```python
from build123d import *

# Parameters (mm, degrees)
SKETCH_R          = 29
PAD_DEPTH         = 35
SKETCH001_W       = 5
SKETCH001_H       = 16
PAD001_DEPTH      = 20
SKETCH002_R       = 4
PAD002_DEPTH      = 66
PAD002_DEPTH_BACK = 48
SKETCH003_R       = 4
SKETCH003_R_2     = 2.4
POCKET_DEPTH      = 20
SKETCH004_R       = 3.25
POCKET001_DEPTH   = 5
FILLET_R          = 2
FILLET001_R       = 7.5


with BuildPart() as part:
    # Sketch → Pad (new body)
    with BuildSketch(Plane.XY):
        Circle(SKETCH_R)
    extrude(amount=PAD_DEPTH)

    # Sketch001 (on Face2 of Pad) → Pad001 (join)
    with BuildSketch(Plane(origin=(0, 0, 0), x_dir=(1, 0, 0), z_dir=(0, 0, -1))):
        Rectangle(SKETCH001_W, SKETCH001_H)
    extrude(amount=PAD001_DEPTH)

    # Sketch002 → Pad002 (join, two sides)
    with BuildSketch(Plane.XZ) as pad002_sk:
        with Locations((0, 8.5)):
            Circle(SKETCH002_R)
    extrude(amount=PAD002_DEPTH)
    extrude(pad002_sk.sketch, amount=-PAD002_DEPTH_BACK)

    # Sketch003 (on Face12 of Pad002) → Pocket (cut)
    with BuildSketch(Plane.XZ.offset(66)):
        with Locations((0, 8.5)):
            Circle(SKETCH003_R)
        with Locations((0, 8.5)):
            Circle(SKETCH003_R_2, mode=Mode.SUBTRACT)
    extrude(amount=-POCKET_DEPTH, mode=Mode.SUBTRACT)

    # Sketch004 (on Face6 of Pocket) → Pocket001 (cut)
    with BuildSketch(Plane.YZ.offset(2.5)):
        with Locations((0, -12)):
            Circle(SKETCH004_R)
    extrude(amount=-POCKET001_DEPTH, mode=Mode.SUBTRACT)

    # Fillet
    fillet_edges = [part.edges().sort_by_distance(p)[0] for p in [
        (-2.4, -66, 8.5),
        (-29, 0, 35),
        (-29, 0, 0),
        (0, 8, 0),
        (0, -8, 0),
        (-4, 48, 8.5),
    ]]
    fillet(fillet_edges, radius=FILLET_R)

    # Fillet001
    fillet001_edges = [part.edges().sort_by_distance(p)[0] for p in [
        (0, -8, -20),
        (0, 8, -20),
    ]]
    fillet(fillet001_edges, radius=FILLET001_R)


solid = part.part
```
The listing builds one solid part. Answer for the finished solid, in the listing's coordinates (mm). A direction names the side the tool comes from. Round coordinates to 2 decimals unless told otherwise and drop trailing zeros. Loops run counter-clockwise (first coordinate to the right, second up) from the corner with the lowest first, then second, coordinate; pieces in that order, holes last.
Q1. Section B-B, the plane z = 18 is taken. Determine the outline of the cut face in (x, y), then the cut area to 3 significant figures.
Q2. Which of the six approach directions +Z, -Z, +X, -X, +Y, -Y give full straight-line access (tool end or side, diameter ignored) to faces 4 (the face through (-0.867, 37.24, 4.595)), 5 (the face through (2.5, 0, -8)), 6 (the face through (-2.5, 0, -8))?
Q3. Section A-A, the plane z = -10.5 is taken. Determine the outline of the cut face in (x, y).
Q4. Find the intervals of material crossed by line 1 (Z direction, x = 0.1, y = 0); line 2 (Z direction, x = 8.5, y = 15.5); line 3 (X direction, y = 37.5, z = 10), in increasing order.
Q5. Given pin 1 Ø10 at (y, z) = (-2.5, -12) entering from -X; pin 2 Ø16 at (y, z) = (4.5, -9.5) entering from +X; pin 3 Ø10 at (y, z) = (9.5, 25) entering from -X, each flat-ended and moving along its own axis, determine where each tip first touches the part or whether it passes through.
Q6. For a pull along Y with two mould halves and no side action, classify faces 1 (the face through (-0.867, -37.24, 4.595)), 2 (the face through (0, 8, -7)), 3 (the face through (0.035, -0.423, -8.778)) as released by +Y, released by -Y, zero draft, split by the parting line, or undercut.
Q7. Section C-C, the plane y = -48 is taken. Determine the outline of the cut face in (x, z), then the cut area to 3 significant figures.
Completed:
1. outline: circle Ø58 at (0, 0)
1. area: 2,640 mm2
2. face 4: +Y
2. face 5: -Z, +X, +Y, -Y
2. face 6: -Z, -X, +Y, -Y
3. outline: (-2.5, -8) - (2.5, -8) - (2.5, -2.88) - (-2.5, -2.88) - close; (-2.5, 2.88) - (2.5, 2.88) - (2.5, 8) - (-2.5, 8) - close
4. line 1: z = -20 to -15.25, -8.75 to 35
4. line 2: z = 0 to 35
4. line 3: x = -3.71 to 3.71
5. pin 1: stops at x = -2.5
5. pin 2: stops at x = 2.5
5. pin 3: stops at x = -28.65
6. face 1: zero draft
6. face 2: released by +Y
6. face 3: undercut
7. outline: circle Ø4.8 at (0, 8.5)
7. area: 18.1 mm2
